```python
from build123d import *

# Parameters (mm, degrees)
SKETCH1_W               = 19.05
SKETCH1_H               = 19.05
SKETCH1_R               = 3.96875
BOSS_EXTRUDE1_DEPTH     = 18.796
CUT_EXTRUDE1_DEPTH      = 33.849575583
CUT_EXTRUDE1_DEPTH_BACK = 33.849575583


with BuildPart() as part:
    # Sketch1 → Boss-Extrude1 (new body)
    with BuildSketch(Plane.XY):
        with Locations((9.525, -9.525)):
            Rectangle(SKETCH1_W, SKETCH1_H)
        with Locations((9.525, -9.525)):
            Circle(SKETCH1_R, mode=Mode.SUBTRACT)
    extrude(amount=-BOSS_EXTRUDE1_DEPTH)

    # Sketch2 → Cut-Extrude1 (cut, two sides: drawn at the far end of the back side and taken through both)
    with BuildSketch(Plane(origin=(0, 0, 0), x_dir=(1, 0, 0), z_dir=(0, 1, 0)).offset(-CUT_EXTRUDE1_DEPTH_BACK)):
        Polygon((0, 7.751616068), (1.6002, 9.398), (0, 11.044383932), align=None)
    extrude(amount=CUT_EXTRUDE1_DEPTH + CUT_EXTRUDE1_DEPTH_BACK, mode=Mode.SUBTRACT)


solid = part.part
```
Read the model definition and answer for the solid it produces. Units are mm, in the model's axes. A direction names the side the tool comes from. Coordinates: 2 decimals unless noted, no trailing zeros. Write each loop counter-clockwise with the first axis right and the second up, starting at its lowest first coordinate (ties: lowest second). Pieces come first, ordered by that corner, then holes. Notation, with made-up numbers: (64.5, -11) -> (81.5, -11) arc R34 cw to (81.5, 28) -> close; hole circle Ø10 at (74, 66.25). An arc over 180 degrees is marked (long way). Write item = value, one per line.
(1) Section B-B on x = 6.25 is taken. Write down the section's boundary in (y, z).
From the geometry:
outline = (-19.05, -18.8) -> (-11.77, -18.8) -> (-11.77, 0) -> (-19.05, 0) -> close; (-7.28, -18.8) -> (0, -18.8) -> (0, 0) -> (-7.28, 0) -> close
(2) Straight lines are drawn through the part: L1, parallel to X at y = -12, z = -5.5; L2, parallel to X at y = -10.5, z = -9.5; L3, parallel to Y at x = 7, z = -13.5. For each, find the intervals that lie inside material, in ascending order. Write a range as from..to.
From the geometry:
L1 = 0..6.42, 12.63..19.05
L2 = 1.5..5.68, 13.37..19.05
L3 = -19.05..-12.59, -6.46..0
(3) For a pull along X with two mould halves and no side action, classify faces 3 (the face through (0.789, -9.658, -8.563)), 4 (the face through (14, -9, 0)), 5 (the face through (8.66, -13.4, -9.27)) as +X half, -X half, draft (parallel to the pull), parting line (faces both ways), or undercut.
From the geometry:
face_3 = -X half
face_4 = draft
face_5 = undercut
(4) Which of the six approach directions +Z, -Z, +X, -X, +Y, -Y give full straight-line access (tool end or side, diameter ignored) to faces 1 (the face through (14, -9, -18.796)), 2 (the face through (0.81, -9.66, -10.21))?
From the geometry:
face_1 = -Z, +X, -X, +Y, -Y
face_2 = -X, +Y, -Y
(5) Section A-A on y = -12.5 is taken. Write down the section's boundary in (x, z).
From the geometry:
outline = (0, -18.8) -> (6.9, -18.8) -> (6.9, 0) -> (0, 0) -> (0, -7.75) -> (1.6, -9.4) -> (0, -11.04) -> close; (12.15, -18.8) -> (19.05, -18.8) -> (19.05, 0) -> (12.15, 0) -> close
(6) Section D-D on y = -8.25 is taken. Write down the section's boundary in (x, z).
From the geometry:
outline = (0, -18.8) -> (5.77, -18.8) -> (5.77, 0) -> (0, 0) -> (0, -7.75) -> (1.6, -9.4) -> (0, -11.04) -> close; (13.28, -18.8) -> (19.05, -18.8) -> (19.05, 0) -> (13.28, 0) -> close
